from build123d import *

# Parameters (mm, degrees)
F0_R          = 16
F0_R_2        = 10
F1_DEPTH      = 3.5
F1_DEPTH_BACK = 3.5
F2_R          = 14.1
F2_R_2        = 11.9
F3_DEPTH      = 0.5


# Not quite as in the source:
# - a pattern or mirror of a feature is missing from the dataset's text; its kind, count and spacing are read off the source's solid


with BuildPart() as f1:
    # F0 (on Front) → F1 (new body, two sides)
    with BuildSketch(Plane.XZ) as f1_sk:
        Circle(F0_R)
        Circle(F0_R_2, mode=Mode.SUBTRACT)
    extrude(amount=F1_DEPTH)
    extrude(f1_sk.sketch, amount=-F1_DEPTH_BACK)

    # F2 (on face) → F3 (cut)
    with BuildSketch(Plane.XZ.offset(3.5)):
        Circle(F2_R)
        Circle(F2_R_2, mode=Mode.SUBTRACT)
    f3 = extrude(amount=-F3_DEPTH, mode=Mode.SUBTRACT)

    # F3_copies: F3 across plane
    add(f3.mirror(Plane.ZX), mode=Mode.SUBTRACT)


solid = f1.part
CAD build for the part. Positions are in the model's coordinates, mm. A direction names the side the tool comes from. Round coordinates to 2 decimals unless told otherwise and drop trailing zeros. Order: outer loops, then holes, each group sorted by start corner. A loop starts at its lowest first (then second) coordinate and runs counter-clockwise, first axis right, second up. Notation, with made-up numbers: (89.25, -38.5) -> (130.25, -38.5) arc R21 cw to (130.25, -31.5) -> close; hole circle Ø6 at (43, 23.25). An arc over 180 degrees is marked (long way). Write item = value, one per line. Start each with the question number.
(1) Pull direction Z, two halves, no side cores. Call faces 1 (the flat face through (6, -3.5, -13)), 2 (the cylindrical face through (-3.47, -0.05, -15.62)), 3 (the cylindrical face through (-8.771, 3.254, 8.043)): released by +Z, released by -Z, zero draft, split by the parting line, or undercut.
(2) Cut at D-D, the plane z = 13. List the corners of the cut face in (x, y).
(3) Cut at C-C, the plane y = 1.25. List the corners of the cut face in (x, z).
(4) Cut at B-B, the plane x = 0. List the corners of the cut face in (y, z), then the cut area to 3 significant figures.
(5) Which spindle directions (+Z, -Z, +X, -X, +Y, -Y) get a long thin tool onto all of the face, cutting with end or side? Do faces 4 (the flat face through (6, 3.5, -13)), 5 (the flat face through (-12, 3, -3)), 6 (the cylindrical face through (-8.771, -3.254, 8.043)). Say none if no direction does.
(6) Cut at A-A, the plane z = 0. List the corners of the cut face in (x, y).
(7) Probe line 1 (Z direction, x = 0, y = -3.05); line 2 (Z direction, x = 0, y = -0.85); line 3 (Z direction, x = -8, y = -2.25). List the from-to ranges inside material, lowest first. Write a range as [from, to].
(8) Pin check, flat tips, straight feed: P1, Ø4, axis at x = -6, y = -2.5, coming from the -Z side; P2, Ø8, axis at x = -3.5, z = -8.5, coming from the +Y side; P3, Ø1.5, axis at x = 2, y = -1, coming from the +Z side; P4, Ø1.5, axis at y = 1, z = -11.5, coming from the +X side. Stop position of each tip, or through.
Model answer:
q1.face_1 = zero draft
q1.face_2 = split by the parting line
q1.face_3 = undercut
q2.outline = (-9.33, -3.5) -> (-5.46, -3.5) -> (-5.46, -3) -> (5.46, -3) -> (5.46, -3.5) -> (9.33, -3.5) -> (9.33, 3.5) -> (5.46, 3.5) -> (5.46, 3) -> (-5.46, 3) -> (-5.46, 3.5) -> (-9.33, 3.5) -> close
q3.outline = circle Ø32 at (0, 0); hole circle Ø20 at (0, 0)
q4.outline = (-3.5, -16) -> (3.5, -16) -> (3.5, -14.1) -> (3, -14.1) -> (3, -11.9) -> (3.5, -11.9) -> (3.5, -10) -> (-3.5, -10) -> (-3.5, -11.9) -> (-3, -11.9) -> (-3, -14.1) -> (-3.5, -14.1) -> close; (-3.5, 10) -> (3.5, 10) -> (3.5, 11.9) -> (3, 11.9) -> (3, 14.1) -> (3.5, 14.1) -> (3.5, 16) -> (-3.5, 16) -> (-3.5, 14.1) -> (-3, 14.1) -> (-3, 11.9) -> (-3.5, 11.9) -> close
q4.area = 79.6 mm2
q5.face_4 = +Z, -Z, +X, -X, +Y
q5.face_5 = +Y
q5.face_6 = -Y
q6.outline = (-16, -3.5) -> (-14.1, -3.5) -> (-14.1, -3) -> (-11.9, -3) -> (-11.9, -3.5) -> (-10, -3.5) -> (-10, 3.5) -> (-11.9, 3.5) -> (-11.9, 3) -> (-14.1, 3) -> (-14.1, 3.5) -> (-16, 3.5) -> close; (10, -3.5) -> (11.9, -3.5) -> (11.9, -3) -> (14.1, -3) -> (14.1, -3.5) -> (16, -3.5) -> (16, 3.5) -> (14.1, 3.5) -> (14.1, 3) -> (11.9, 3) -> (11.9, 3.5) -> (10, 3.5) -> close
q7.line_1 = [-16, -14.1], [-11.9, -10], [10, 11.9], [14.1, 16]
q7.line_2 = [-16, -10], [10, 16]
q7.line_3 = [-13.86, -6], [6, 13.86]
q8.P1 = -15.49
q8.P2 = 3.5
q8.P3 = 15.95
q8.P4 = 11.85
